```python
from build123d import *

# Parameters (mm, degrees)
SKETCH_1_W             = 60
SKETCH_1_H             = 60
EXTRUDE_1_DEPTH        = 12
HOLE_WIZARD_M161_D     = 14
HOLE_WIZARD_M161_DEPTH = 12
SKETCH_12_R            = 4.5
CUT_EXTRUDE_1_DEPTH    = 13
SKETCH_13_R            = 7.5
CUT_EXTRUDE_2_DEPTH    = 9


with BuildPart() as part:
    # Эскиз1 → Бобышка-Вытянуть1 (new body)
    with BuildSketch(Plane(origin=(0, 0, 0), x_dir=(1, 0, 0), z_dir=(0, 1, 0))):
        Rectangle(SKETCH_1_W, SKETCH_1_H)
    extrude(amount=EXTRUDE_1_DEPTH)

    # Отверстие обработанное метчиком M161
    with Locations(Plane(origin=(0, 12, 0), x_dir=(1, 0, 0), z_dir=(0, 1, 0))):
        with Locations((0, 0)):
            Hole(HOLE_WIZARD_M161_D / 2, depth=HOLE_WIZARD_M161_DEPTH)

    # Эскиз12 → Вырез-Вытянуть1 (cut, through all)
    with BuildSketch(Plane(origin=(0, 12, 0), x_dir=(1, 0, 0), z_dir=(0, 1, 0))):
        with Locations(Location((-15, 15, 0), (0, 0, 270))):  # turned: the seam where the file's is
            Circle(SKETCH_12_R)
        with Locations(Location((15, 15, 0), (0, 0, 270))):  # turned: the seam where the file's is
            Circle(SKETCH_12_R)
        with Locations(Location((15, -15, 0), (0, 0, 270))):  # turned: the seam where the file's is
            Circle(SKETCH_12_R)
        with Locations(Location((-15, -15, 0), (0, 0, 270))):  # turned: the seam where the file's is
            Circle(SKETCH_12_R)
    extrude(amount=-CUT_EXTRUDE_1_DEPTH, mode=Mode.SUBTRACT)

    # Эскиз13 → Вырез-Вытянуть2 (cut)
    with BuildSketch(Plane(origin=(0, 12, 0), x_dir=(1, 0, 0), z_dir=(0, 1, 0))):
        with Locations(Location((-15, 15, 0), (0, 0, 270))):  # turned: the seam where the file's is
            Circle(SKETCH_13_R)
        with Locations(Location((15, 15, 0), (0, 0, 270))):  # turned: the seam where the file's is
            Circle(SKETCH_13_R)
        with Locations(Location((15, -15, 0), (0, 0, 270))):  # turned: the seam where the file's is
            Circle(SKETCH_13_R)
        with Locations(Location((-15, -15, 0), (0, 0, 270))):  # turned: the seam where the file's is
            Circle(SKETCH_13_R)
    extrude(amount=-CUT_EXTRUDE_2_DEPTH, mode=Mode.SUBTRACT)


solid = part.part
```
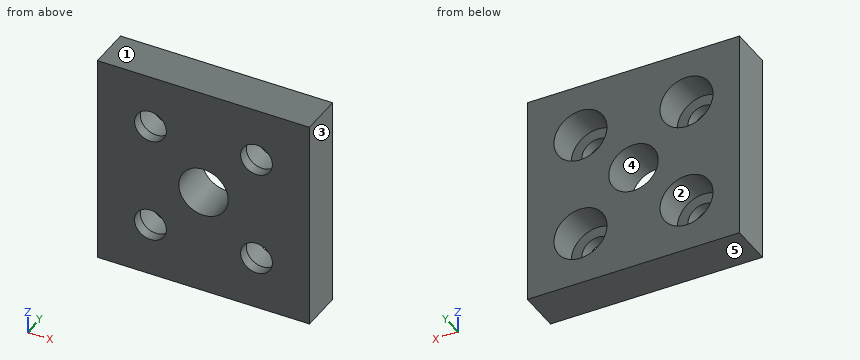
CAD build for the part. Positions are in the model's coordinates, mm. Face numbers are marked on the shaded views. A direction names the side the tool comes from. Give positions to 0.01 mm unless a question says otherwise; leave off trailing zeros. Order: outer loops, then holes, each group sorted by start corner. A loop starts at its lowest first (then second) coordinate and runs counter-clockwise, first axis right, second up.
(1) Tool access for the marked faces 1 and 2: list every direction of +Z, -Z, +X, -X, +Y, -Y with a clear straight run to the whole face (end or side of a thin tool).
(2) Drill centre lines: L1, parallel to Z at x = -21, y = 5; L2, parallel to Z at x = -14.5, y = 6.25. Where is each one in solid material? Low to high.
(3) Saw through at A-A, the plane z = 0. Give the cut face in (x, y), then the cut area to 3 significant figures.
(4) Mould opens along Z. For the marked faces 3, 4 and 5 say: released by +Z, released by -Z, zero draft, split by the parting line, or undercut.
(5) Saw through at D-D, the plane x = 15. Give the cut face in (y, z), then the cut area to 3 significant figures.
(6) Saw through at C-C, the plane z = -15. Give the cut face in (x, y).
(7) Saw through at B-B, the plane y = 1.5. Give the cut face in (x, z), then the cut area to 3 significant figures.
(8) Flat gauge pins, fed straight in: pin 1 (7.5 mm diameter, centred on x = 17.5, z = 15, fed in from +Y); pin 2 (19.5 mm diameter, centred on x = -15, z = 15, fed in from -Y). Where does each tip first touch, or does it go through?
Results found:
1. face 1: +Z, +X, -X, +Y, -Y
1. face 2: +Y
2. L1: z = -30 to -19.5, -10.5 to 10.5, 19.5 to 30
2. L2: z = -30 to -22.48, -7.52 to 7.52, 22.48 to 30
3. outline: (-30, 0) - (-7, 0) - (-7, 12) - (-30, 12) - close; (7, 0) - (30, 0) - (30, 12) - (7, 12) - close
3. area: 552 mm2
4. face 3: zero draft
4. face 4: undercut
4. face 5: released by -Z
5. outline: (0, -30) - (12, -30) - (12, -22.5) - (3, -22.5) - (3, -19.5) - (0, -19.5) - close; (0, -10.5) - (3, -10.5) - (3, -7.5) - (12, -7.5) - (12, 7.5) - (3, 7.5) - (3, 10.5) - (0, 10.5) - close; (0, 19.5) - (3, 19.5) - (3, 22.5) - (12, 22.5) - (12, 30) - (0, 30) - close
5. area: 396 mm2
6. outline: (-30, 0) - (-19.5, 0) - (-19.5, 3) - (-22.5, 3) - (-22.5, 12) - (-30, 12) - close; (-10.5, 0) - (10.5, 0) - (10.5, 3) - (7.5, 3) - (7.5, 12) - (-7.5, 12) - (-7.5, 3) - (-10.5, 3) - close; (19.5, 0) - (30, 0) - (30, 12) - (22.5, 12) - (22.5, 3) - (19.5, 3) - close
7. outline: (-30, -30) - (30, -30) - (30, 30) - (-30, 30) - close; hole circle Ø9 at (-15, -15); hole circle Ø9 at (-15, 15); hole circle Ø14 at (0, 0); hole circle Ø9 at (15, -15); hole circle Ø9 at (15, 15)
7. area: 3,190 mm2
8. pin 1: stops at y = 3
8. pin 2: stops at y = 0
